from build123d import *

# Parameters (mm, degrees)
BOSS_EXTRUDE1_DEPTH                                 = 6
SKETCH3_W                                           = 53.5
SKETCH3_H                                           = 8
BOSS_EXTRUDE2_DEPTH                                 = 2
CSK_FOR_M3_COUNTERSUNK_FLAT_HEAD_SCREW1_D           = 3.6
CSK_FOR_M3_COUNTERSUNK_FLAT_HEAD_SCREW1_CSINK_D     = 6.3
CSK_FOR_M3_COUNTERSUNK_FLAT_HEAD_SCREW1_CSINK_ANGLE = 90
CUT_EXTRUDE1_DEPTH                                  = 29.66727228
BOSS_EXTRUDE3_DEPTH                                 = 8
SKETCH8_W                                           = 24
SKETCH8_H                                           = 1.5
BOSS_EXTRUDE4_DEPTH                                 = 2
CSK_FOR_M3_COUNTERSUNK_FLAT_HEAD_SCREW2_D           = 3.6
CSK_FOR_M3_COUNTERSUNK_FLAT_HEAD_SCREW2_CSINK_D     = 6.3
CSK_FOR_M3_COUNTERSUNK_FLAT_HEAD_SCREW2_CSINK_ANGLE = 90


with BuildPart() as part:
    # Sketch1 → Boss-Extrude1 (new body)
    with BuildSketch(Plane.XY):
        Polygon((-18, 0), (-18, 6.5), (-26.75, 6.5), (-26.75, -1.5), (26.75, -1.5), (26.75, 6.5), (18, 6.5), (18, 0), align=None)
    extrude(amount=BOSS_EXTRUDE1_DEPTH)

    # Sketch3 → Boss-Extrude2 (add)
    with BuildSketch(Plane.XY.offset(6)):
        with Locations((0, 2.5)):
            Rectangle(SKETCH3_W, SKETCH3_H)
    extrude(amount=BOSS_EXTRUDE2_DEPTH)

    # CSK for M3 Countersunk Flat Head Screw1 (through all)
    with Locations(Plane(origin=(0, -1.5, 0), x_dir=(-1, 0, 0), z_dir=(0, -1, 0))):
        with Locations((0, -3)):
            CounterSinkHole(CSK_FOR_M3_COUNTERSUNK_FLAT_HEAD_SCREW1_D / 2, CSK_FOR_M3_COUNTERSUNK_FLAT_HEAD_SCREW1_CSINK_D / 2, counter_sink_angle=CSK_FOR_M3_COUNTERSUNK_FLAT_HEAD_SCREW1_CSINK_ANGLE)

    # Sketch6 → Cut-Extrude1 (cut, through all)
    with BuildSketch(Plane(origin=(0, 0, 0), x_dir=(1, 0, 0), z_dir=(0, 1, 0))):
        with BuildLine():
            Line((16, 0), (16, -3))
            ThreePointArc((16, -3), (14, -5), (12, -3))
            Line((12, -3), (12, 0))
            ThreePointArc((12, 0), (14, 2), (16, 0))
        make_face()
        with BuildLine():
            Line((-16, 0), (-16, -3))
            ThreePointArc((-16, -3), (-14, -5), (-12, -3))
            Line((-12, -3), (-12, 0))
            ThreePointArc((-12, 0), (-14, 2), (-16, 0))
        make_face()
    extrude(amount=-CUT_EXTRUDE1_DEPTH, mode=Mode.SUBTRACT)

    # Sketch7 → Boss-Extrude3 (add, through all)
    with BuildSketch(Plane(origin=(0, -1.5, 0), x_dir=(1, 0, 0), z_dir=(0, 1, 0))):
        with BuildLine():
            Line((26.75, -12), (26.75, -8))
            Line((26.75, -8), (-26.75, -8))
            Line((-26.75, -8), (-26.75, -12))
            ThreePointArc((-26.75, -12), (0, -9.420658927), (26.75, -12))
        make_face()
    extrude(amount=BOSS_EXTRUDE3_DEPTH)

    # Sketch8 → Boss-Extrude4 (add)
    with BuildSketch(Plane(origin=(0, 0, 0), x_dir=(-1, 0, 0), z_dir=(0, 0, -1))):
        Polygon((-26.75, 6.5), (-18, 6.5), (-18, 0), (-16, 0), (-16, -1.5), (-26.75, -1.5), align=None)
        with Locations((0, -0.75)):
            Rectangle(SKETCH8_W, SKETCH8_H)
        Polygon((18, 6.5), (26.75, 6.5), (26.75, -1.5), (16, -1.5), (16, 0), (18, 0), align=None)
    extrude(amount=BOSS_EXTRUDE4_DEPTH)

    # CSK for M3 Countersunk Flat Head Screw2 (through all)
    with Locations(Plane(origin=(0, -1.5, 0), x_dir=(-1, 0, 0), z_dir=(0, -1, 0))):
        with Locations((0, -3)):
            CounterSinkHole(CSK_FOR_M3_COUNTERSUNK_FLAT_HEAD_SCREW2_D / 2, CSK_FOR_M3_COUNTERSUNK_FLAT_HEAD_SCREW2_CSINK_D / 2, counter_sink_angle=CSK_FOR_M3_COUNTERSUNK_FLAT_HEAD_SCREW2_CSINK_ANGLE)


solid = part.part
Could you check a few things on this model? Use its own coordinates, in mm. A direction names the side the tool comes from. Coordinates: 2 decimals unless noted, no trailing zeros. Loops run counter-clockwise (first coordinate to the right, second up) from the corner with the lowest first, then second, coordinate; pieces in that order, holes last.
1. For faces 1 (the face through (-16, -1, 0)), 2 (the face through (0, -1.5, 7)), 3 (the face through (18, 3, 2)), which set-ups out of +Z, -Z, +X, -X, +Y, -Y let a thin tool reach every point of the face, with its end or its side?
2. For P1, Ø1.5, axis at x = 21.5, y = 3, coming from the +Z side; P2, Ø4, axis at x = -5, z = 2, coming from the +Y side; P3, Ø2, axis at x = -7.5, y = 3, coming from the +Z side, each with a flat end and sliding along its axis, tell me the tip position at first contact or that it passes through.
3. I need wall thicknesses on L1, parallel to Z at x = 0, y = -0.05; L2, parallel to X at y = 5.5, z = 2.5; L3, parallel to Y at x = -9, z = 3. Which ranges of each line are inside material? Lowest first, please.
4. Imagine slicing it at D-D (x = -14). Please give me the cut outline in (y, z), and give its area (3 significant figures).
5. Imagine slicing it at B-B (y = 2). Please give me the cut outline in (x, z), and give its area (3 significant figures).
6. We'd pull the mould along X, two halves only. Please class faces 4 (the face through (0, -1, -2)), 5 (the face through (-18, 3, 2)), 6 (the face through (26.75, 2, 5)): released by +X, released by -X, zero draft, split by the parting line, or undercut.
7. Imagine slicing it at A-A (x = 0). Please give me the cut outline in (y, z), and give its area (3 significant figures).
Computed values:
1. face 1: -Z, +Y, -Y
1. face 2: +Z, -Z, +X, -X, -Y
1. face 3: -Z, +Y
2. P1: stops at z = 11.2
2. P2: stops at y = 0
2. P3: stops at z = 9.68
3. L1: z = -2 to 1.2, 4.8 to 9.42
3. L2: x = -26.75 to -18, 18 to 26.75
3. L3: y = -1.5 to 0
4. outline: (-1.5, 5) - (0, 5) - (0, 6) - (6.5, 6) - (6.5, 10.12) - (-1.5, 10.12) - close
4. area: 34.5 mm2
5. outline: (-26.75, -2) - (-18, -2) - (-18, 6) - (18, 6) - (18, -2) - (26.75, -2) - (26.75, 12) arc R140 cw to (-26.75, 12) - close
5. area: 369 mm2
6. face 4: zero draft
6. face 5: undercut
6. face 6: released by +X
7. outline: (-1.5, -2) - (0, -2) - (0, 1.2) - (-0.15, 1.2) - (-1.5, -0.15) - close; (-1.5, 6.15) - (-0.15, 4.8) - (0, 4.8) - (0, 6) - (6.5, 6) - (6.5, 9.42) - (-1.5, 9.42) - close
7. area: 32.1 mm2
